```python
from build123d import *

# Parameters (mm, degrees)
EXTRUDE_1_DEPTH   = 10
FILLET_1_R        = 1
HOLE_WIZARD_M41_D = 4.5
M4X0_71_D         = 3.3


with BuildPart() as part:
    # Эскиз2 → Бобышка-Вытянуть1 (new body)
    with BuildSketch(Plane(origin=(0, 382.645061039, 0), x_dir=(1, 0, 0), z_dir=(0, 1, 0))):
        with BuildLine():
            Line((3.565848943, 102.673881836), (3.565848943, 110.773881836))
            Line((3.565848943, 110.773881836), (14.565848943, 110.773881836))
            Line((14.565848943, 110.773881836), (14.565848943, 50.773881836))
            Line((14.565848943, 50.773881836), (3.565848943, 50.773881836))
            Line((3.565848943, 50.773881836), (3.565848943, 58.873881836))
            ThreePointArc((3.565848943, 58.873881836), (10.565848943, 65.873881836), (3.565848943, 72.873881836))
            Line((3.565848943, 72.873881836), (3.565848943, 88.673881836))
            ThreePointArc((3.565848943, 88.673881836), (10.565848943, 95.673881836), (3.565848943, 102.673881836))
        make_face()
    extrude(amount=-EXTRUDE_1_DEPTH)

    # Скругление1
    fillet_1_edges = [part.edges().sort_by_distance(p)[0] for p in [
        (3.565848943, 377.645061039, -50.773881836),
        (3.565848943, 377.645061039, -110.773881836),
    ]]
    fillet(fillet_1_edges, radius=FILLET_1_R)

    # Отверстие с зазором M41 (through all)
    with Locations(Plane(origin=(3.565848943, 346.946860721, -25.652823237), x_dir=(0, 0, 1), z_dir=(-1, 0, 0))):
        with Locations((-80.8710586, 30.698200318), (-29.3710586, 30.698200318)):
            Hole(HOLE_WIZARD_M41_D / 2)

    # Отверстие обработанное метчиком M4x0.71 (through all)
    with Locations(Plane(origin=(3.565848943, 346.946860721, -25.652823237), x_dir=(0, 0, 1), z_dir=(-1, 0, 0))):
        with Locations((-55.1210586, 30.698200318)):
            Hole(M4X0_71_D / 2)


solid = part.part
```
For this review, take the finished solid that the model builds, in its own axes (mm). Give positions to 0.01 mm unless a question says otherwise; leave off trailing zeros. Loops run counter-clockwise (first coordinate to the right, second up) from the corner with the lowest first, then second, coordinate; pieces in that order, holes last. Notation, with made-up numbers: M 72.25,35 L 106.25,35 A14 cw 106.25,51 Z; hole C 41,40.25 d8. An arc over 180 degrees is marked long. One line per item, written item: value. Start each with the question number.
Q1. Add section C-C (y = 373.75). Give the boundary of the cut face in (x, z).
Q2. Add section A-A (x = 6.5). Give the boundary of the cut face in (y, z), and give its area (3 significant figures).
Q3. Add section B-B (z = -105). Give the boundary of the cut face in (x, y).
Q4. Draft analysis for pull direction Y (two halves, no side actions). For faces 1 (the face through (9, 378, -110.774)), 2 (the face through (9.143, 376.276, -104.738)), 3 (the face through (10, 372.645, -81)), state which applies: released by +Y, released by -Y, zero draft, split by the parting line, or undercut.
Q5. For L1, parallel to Z at x = 8, y = 379; L2, parallel to Z at x = 6, y = 374.75; L3, parallel to Z at x = 6.75, y = 382, list the stretches that pass through material, from the lowest coordinate up.
Q6. Add section D-D (y = 378.5). Give the boundary of the cut face in (x, z), and give its area (3 significant figures).
Reply:
1. outline: M 3.57,-109.77 A1 ccw 4.57,-110.77 L 14.57,-110.77 L 14.57,-50.77 L 4.57,-50.77 A1 ccw 3.57,-51.77 L 3.57,-58.87 A7 cw 3.57,-72.87 L 3.57,-88.67 A7 cw 3.57,-102.67 Z
2. outline: M 372.65,-110.77 L 382.65,-110.77 L 382.65,-102.03 L 372.65,-102.03 Z; M 372.65,-89.32 L 382.65,-89.32 L 382.65,-72.23 L 372.65,-72.23 Z; M 372.65,-59.52 L 382.65,-59.52 L 382.65,-50.77 L 372.65,-50.77 Z; hole C 377.65,-106.52 d4.5; hole C 377.65,-55.02 d4.5; hole C 377.65,-80.77 d3.3
2. area: 305 mm²
3. outline: M 3.57,372.65 L 14.57,372.65 L 14.57,375.99 L 3.57,375.99 Z; M 3.57,379.3 L 14.57,379.3 L 14.57,382.65 L 3.57,382.65 Z
4. face 1: zero draft
4. face 2: undercut
4. face 3: released by -Y
5. L1: -110.77 to -108.32, -104.73 to -101.09, -90.26 to -81.72, -79.83 to -71.29, -60.46 to -56.82, -53.23 to -50.77
5. L2: -110.77 to -102.24, -89.11 to -72.44, -59.31 to -50.77
5. L3: -110.77 to -101.91, -89.44 to -72.11, -59.64 to -50.77
6. outline: M 3.57,-109.77 A1 ccw 4.57,-110.77 L 14.57,-110.77 L 14.57,-108.61 L 3.57,-108.61 Z; M 3.57,-104.44 L 14.57,-104.44 L 14.57,-82.19 L 3.57,-82.19 L 3.57,-88.67 A7 cw 3.57,-102.67 Z; M 3.57,-79.36 L 14.57,-79.36 L 14.57,-57.11 L 3.57,-57.11 L 3.57,-58.87 A7 cw 3.57,-72.87 Z; M 3.57,-52.94 L 14.57,-52.94 L 14.57,-50.77 L 4.57,-50.77 A1 ccw 3.57,-51.77 Z
6. area: 383 mm²
